from build123d import *

# Parameters (mm, degrees)
SKETCH1_W                  = 69.26
SKETCH1_H                  = 52.26
BOSS_EXTRUDE3_DEPTH        = 29.208
SKETCH2_W                  = 59.1
SKETCH2_H                  = 42.1
CUT_EXTRUDE4_DEPTH         = 24.128
FILLET1_R                  = 5
SKETCH3_R                  = 4.8067
BOSS_EXTRUDE4_DEPTH        = 11.43
SKETCH3_3_R                = 2.8067
CUT_EXTRUDE5_DEPTH         = 6.35
SKETCH9_R                  = 4.8067
SKETCH9_R_2                = 2.8067
BOSS_EXTRUDE5_DEPTH        = 6.35
SKETCH10_R                 = 2.159
CUT_EXTRUDE6_DEPTH         = 5.08
BOSS_EXTRUDE6_DEPTH        = 1
FACE_2_CONNECTOR_HOLES_W   = 6.4
FACE_2_CONNECTOR_HOLES_H   = 5
FACE_2_CONNECTOR_HOLES_W_2 = 10.4
CUT_EXTRUDE7_DEPTH         = 5.08
FACE_3_CONNECTOR_HOLES_W   = 6.4
FACE_3_CONNECTOR_HOLES_H   = 5
CUT_EXTRUDE8_DEPTH         = 5.08
FACE_4_CONNECTOR_HOLES_W   = 34.7
FACE_4_CONNECTOR_HOLES_H   = 5
CUT_EXTRUDE9_DEPTH         = 5.08


with BuildPart() as part:
    # Sketch1 → Boss-Extrude3 (new body)
    with BuildSketch(Plane(origin=(0, 0, 0), x_dir=(1, 0, 0), z_dir=(0, 1, 0))):
        Rectangle(SKETCH1_W, SKETCH1_H)
    extrude(amount=BOSS_EXTRUDE3_DEPTH)

    # Sketch2 → Cut-Extrude4 (cut)
    with BuildSketch(Plane(origin=(0, 29.208, 0), x_dir=(1, 0, 0), z_dir=(0, 1, 0))):
        Rectangle(SKETCH2_W, SKETCH2_H)
    extrude(amount=-CUT_EXTRUDE4_DEPTH, mode=Mode.SUBTRACT)

    # Fillet1
    fillet1_edges = [part.edges().sort_by_distance(p)[0] for p in [
        (-34.63, 14.604, 26.13),
        (34.63, 14.604, 26.13),
        (34.63, 14.604, -26.13),
        (-34.63, 14.604, -26.13),
    ]]
    fillet(fillet1_edges, radius=FILLET1_R)

    # Sketch3 → Boss-Extrude4 (add)
    with BuildSketch(Plane(origin=(0, 29.208, 0), x_dir=(1, 0, 0), z_dir=(0, 1, 0))):
        with Locations((-29.55, 21.05)):
            Circle(SKETCH3_R)
        with Locations((29.55, 21.05)):
            Circle(SKETCH3_R)
        with Locations((-29.55, -21.05)):
            Circle(SKETCH3_R)
        with Locations((29.55, -21.05)):
            Circle(SKETCH3_R)
    extrude(amount=-BOSS_EXTRUDE4_DEPTH)

    # Sketch3<3> → Cut-Extrude5 (cut)
    with BuildSketch(Plane(origin=(0, 29.208, 0), x_dir=(1, 0, 0), z_dir=(0, 1, 0))):
        with Locations(Location((-29.55, 21.05, 0), (0, 0, 270))):
            Circle(SKETCH3_3_R)
        with Locations(Location((29.55, 21.05, 0), (0, 0, 270))):
            Circle(SKETCH3_3_R)
        with Locations(Location((29.55, -21.05, 0), (0, 0, 270))):
            Circle(SKETCH3_3_R)
        with Locations(Location((-29.55, -21.05, 0), (0, 0, 270))):
            Circle(SKETCH3_3_R)
    extrude(amount=-CUT_EXTRUDE5_DEPTH, mode=Mode.SUBTRACT)

    # Sketch9 → Boss-Extrude5 (add)
    # profile 1 of 4: a face of its own
    with BuildSketch(Plane(origin=(0, 5.08, 0), x_dir=(1, 0, 0), z_dir=(0, 1, 0))):
        with Locations(Location((-23.35, 14.9, 0), (0, 0, 90))):
            Circle(SKETCH9_R)
        with Locations(Location((-23.35, 14.9, 0), (0, 0, 270))):
            Circle(SKETCH9_R_2, mode=Mode.SUBTRACT)
    # profile 2 of 4: a face of its own
    with BuildSketch(Plane(origin=(0, 5.08, 0), x_dir=(1, 0, 0), z_dir=(0, 1, 0))):
        with Locations(Location((23.65, 15.15, 0), (0, 0, 90))):
            Circle(SKETCH9_R)
        with Locations(Location((23.65, 15.15, 0), (0, 0, 270))):
            Circle(SKETCH9_R_2, mode=Mode.SUBTRACT)
    # profile 3 of 4: a face of its own
    with BuildSketch(Plane(origin=(0, 5.08, 0), x_dir=(1, 0, 0), z_dir=(0, 1, 0))):
        with Locations(Location((23.4, -15.1, 0), (0, 0, 90))):
            Circle(SKETCH9_R)
        with Locations(Location((23.4, -15.1, 0), (0, 0, 270))):
            Circle(SKETCH9_R_2, mode=Mode.SUBTRACT)
    # profile 4 of 4: a face of its own
    with BuildSketch(Plane(origin=(0, 5.08, 0), x_dir=(1, 0, 0), z_dir=(0, 1, 0))):
        with Locations(Location((-23.6, -15.1, 0), (0, 0, 90))):
            Circle(SKETCH9_R)
        with Locations(Location((-23.6, -15.1, 0), (0, 0, 270))):
            Circle(SKETCH9_R_2, mode=Mode.SUBTRACT)
    extrude(amount=BOSS_EXTRUDE5_DEPTH)

    # Sketch10 → Cut-Extrude6 (cut)
    with BuildSketch(Plane(origin=(0, 5.08, 0), x_dir=(1, 0, 0), z_dir=(0, 1, 0))):
        with Locations(Location((14.275, 10.025, 0), (0, 0, 270))):
            Circle(SKETCH10_R)
        with Locations(Location((14.275, -10.025, 0), (0, 0, 270))):
            Circle(SKETCH10_R)
        with Locations(Location((-14.275, 10.025, 0), (0, 0, 270))):
            Circle(SKETCH10_R)
        with Locations(Location((-14.275, -10.025, 0), (0, 0, 270))):
            Circle(SKETCH10_R)
    extrude(amount=-CUT_EXTRUDE6_DEPTH, mode=Mode.SUBTRACT)

    # Sketch12 → Boss-Extrude6 (add)
    with BuildSketch(Plane(origin=(0, 5.08, 0), x_dir=(1, 0, 0), z_dir=(0, 1, 0))):
        Polygon((-26.671494391, 9.324758956), (-26.024358974, 9.324758956), (-26.024358974, 5.824758956), (-26.338461538, 5.824758956), (-26.338461538, 8.965784597), (-26.876923077, 8.965784597), align=None)
    extrude(amount=BOSS_EXTRUDE6_DEPTH)

    # Face 2 Connector Holes → Cut-Extrude7 (cut)
    with BuildSketch(Plane(origin=(0, 0, -26.13), x_dir=(-1, 0, 0), z_dir=(0, 0, -1))):
        with Locations((15.03, 15.53)):
            Rectangle(FACE_2_CONNECTOR_HOLES_W, FACE_2_CONNECTOR_HOLES_H)
        with Locations((-13.27, 15.53)):
            Rectangle(FACE_2_CONNECTOR_HOLES_W_2, FACE_2_CONNECTOR_HOLES_H)
    extrude(amount=-CUT_EXTRUDE7_DEPTH, mode=Mode.SUBTRACT)

    # Face 3 Connector Holes → Cut-Extrude8 (cut)
    with BuildSketch(Plane(origin=(34.63, 0, 0), x_dir=(0, 0, -1), z_dir=(1, 0, 0))):
        with Locations((6.88, 15.53)):
            Rectangle(FACE_3_CONNECTOR_HOLES_W, FACE_3_CONNECTOR_HOLES_H)
    extrude(amount=-CUT_EXTRUDE8_DEPTH, mode=Mode.SUBTRACT)

    # Face 4 Connector Holes → Cut-Extrude9 (cut)
    with BuildSketch(Plane.XY.offset(26.13)):
        with Locations((0.08, 15.53)):
            Rectangle(FACE_4_CONNECTOR_HOLES_W, FACE_4_CONNECTOR_HOLES_H)
    extrude(amount=-CUT_EXTRUDE9_DEPTH, mode=Mode.SUBTRACT)


solid = part.part
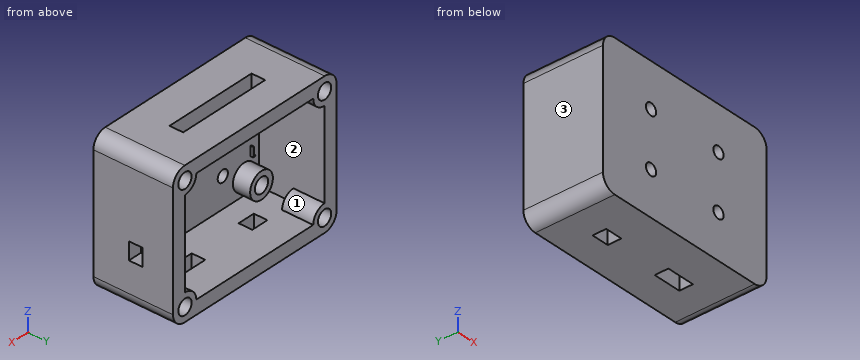
Source: CAD feature listing. Evaluate the final solid. Frame: model axes, mm. Face numbers are marked on the shaded views. A direction names the side the tool comes from. Coordinates: 2 decimals unless noted, no trailing zeros. Order: outer loops, then holes, each group sorted by start corner. A loop starts at its lowest first (then second) coordinate and runs counter-clockwise, first axis right, second up.
Item 1: Cut plane B-B (x = -9.5). Return loops of the section in (y, z), plus the area to 3 significant figures.
Output values:
outline: (0, -26.13) - (29.21, -26.13) - (29.21, -21.05) - (5.08, -21.05) - (5.08, 21.05) - (13.03, 21.05) - (13.03, 26.13) - (0, 26.13) - close; (18.03, 21.05) - (29.21, 21.05) - (29.21, 26.13) - (18.03, 26.13) - close
area: 485 mm2
Item 2: Cut plane D-D (z = 15.1). Return loops of the section in (x, y), plus the area to 3 significant figures.
Output values:
outline: (-34.63, 0) - (34.63, 0) - (34.63, 29.21) - (29.55, 29.21) - (29.55, 5.08) - (28.21, 5.08) - (28.21, 11.43) - (26.21, 11.43) - (26.21, 5.08) - (20.59, 5.08) - (20.59, 11.43) - (18.59, 11.43) - (18.59, 5.08) - (-18.79, 5.08) - (-18.79, 11.43) - (-20.79, 11.43) - (-20.79, 5.08) - (-26.41, 5.08) - (-26.41, 11.43) - (-28.41, 11.43) - (-28.41, 5.08) - (-29.55, 5.08) - (-29.55, 29.21) - (-34.63, 29.21) - close
area: 648 mm2
Item 3: Material intervals for line 1 (X direction, y = 6.5, z = 15.1); line 2 (X direction, y = 6.75, z = -14.9); line 3 (X direction, y = 6, z = -8.5), sorted ascending.
Output values:
line 1: x = -34.63 to -29.55, -28.41 to -26.41, -20.79 to -18.79, 18.59 to 20.59, 26.21 to 28.21, 29.55 to 34.63
line 2: x = -34.63 to -29.55, -28.16 to -26.16, -20.54 to -18.54, 18.85 to 20.85, 26.45 to 28.45, 29.55 to 34.63
line 3: x = -34.63 to -29.55, -26.34 to -26.02, 29.55 to 34.63
Item 4: Cut plane C-C (z = -1). Return loops of the section in (x, y), plus the area to 3 significant figures.
Output values:
outline: (-34.63, 0) - (34.63, 0) - (34.63, 29.21) - (29.55, 29.21) - (29.55, 5.08) - (-29.55, 5.08) - (-29.55, 29.21) - (-34.63, 29.21) - close
area: 597 mm2
Item 5: Set-up query: the marked faces 1, 2 and 3. Return all of +Z, -Z, +X, -X, +Y, -Y with unobstructed straight access to the full face (end or side cutting, diameter ignored); none if empty.
Output values:
face 1: +Y
face 2: none
face 3: +Z, -Z, -X, +Y, -Y
Item 6: Cut plane A-A (y = 20.25). Return loops of the section in (x, z).
Output values:
outline: (-34.63, -21.13) arc R5 ccw to (-29.63, -26.13) - (29.63, -26.13) arc R5 ccw to (34.63, -21.13) - (34.63, 21.13) arc R5 ccw to (29.63, 26.13) - (-29.63, 26.13) arc R5 ccw to (-34.63, 21.13) - close; hole (-29.55, -16.24) arc R4.81 cw to (-24.74, -21.05) - (24.74, -21.05) arc R4.81 cw to (29.55, -16.24) - (29.55, 16.24) arc R4.81 cw to (24.74, 21.05) - (-24.74, 21.05) arc R4.81 cw to (-29.55, 16.24) - close
Item 7: First-contact query: P1, Ø5.5, axis at x = -14.275, z = 10.025, coming from the +Y side; P2, Ø5, axis at x = 7.5, y = 13.5, coming from the +Z side; P3, Ø5.5, axis at y = 14.5, z = -24.5, coming from the -X side; P4, Ø1.5, axis at x = 31.5, y = 14.5, coming from the -Z side. Flat tips, straight axial feed; report the tip coordinate or a pass-through.
Output values:
P1: stops at y = 5.08
P2: stops at z = 26.13
P3: stops at x = -34.59
P4: stops at z = -26
